The listing builds one solid part. Answer for the finished solid, in the listing's coordinates (mm). Face numbers are marked on the shaded views. A direction names the side the tool comes from. Give positions to 0.01 mm unless a question says otherwise; leave off trailing zeros. Loops run counter-clockwise (first coordinate to the right, second up) from the corner with the lowest first, then second, coordinate; pieces in that order, holes last. Notation, with made-up numbers: M 56,2 L 112,2 A26 cw 112,27 Z; hole C 87,72.5 d10. An arc over 180 degrees is marked long. Return JSON: item names as keys, results as strings.
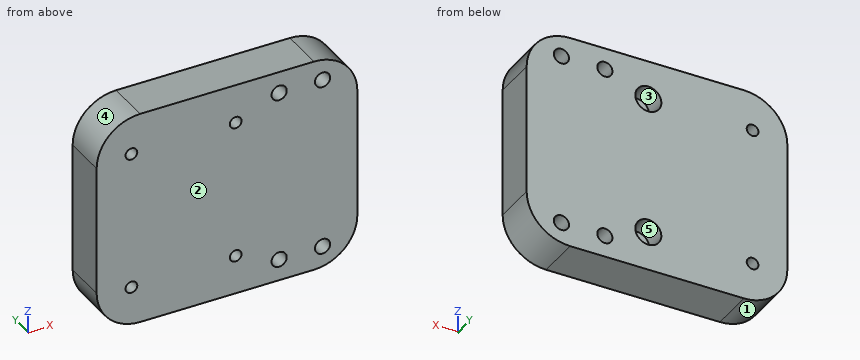
from build123d import *

# Parameters (mm, degrees)
SKETCH1_W           = 60
SKETCH1_H           = 50
BOSS_EXTRUDE1_DEPTH = 10
SKETCH2_R           = 1.35
CUT_EXTRUDE1_DEPTH  = 79.74007874
SKETCH3_R           = 1.75
CUT_EXTRUDE2_DEPTH  = 79.74007874
FILLET1_R           = 10
SKETCH4_R           = 3
CUT_EXTRUDE3_DEPTH  = 5


with BuildPart() as part:
    # Sketch1 → Boss-Extrude1 (new body)
    with BuildSketch(Plane(origin=(0, 0, 0), x_dir=(1, 0, 0), z_dir=(0, 1, 0))):
        with Locations((30, 25)):
            Rectangle(SKETCH1_W, SKETCH1_H)
    extrude(amount=BOSS_EXTRUDE1_DEPTH)

    # Sketch2 → Cut-Extrude1 (cut, through all)
    with BuildSketch(Plane(origin=(0, 10, 0), x_dir=(1, 0, 0), z_dir=(0, 1, 0))):
        with Locations(Location((8, 41, 0), (0, 0, 270))):
            Circle(SKETCH2_R)
        with Locations(Location((8, 9, 0), (0, 0, 270))):
            Circle(SKETCH2_R)
        with Locations(Location((32, 9, 0), (0, 0, 270))):
            Circle(SKETCH2_R)
        with Locations(Location((32, 41, 0), (0, 0, 270))):
            Circle(SKETCH2_R)
    extrude(amount=-CUT_EXTRUDE1_DEPTH, mode=Mode.SUBTRACT)

    # Sketch3 → Cut-Extrude2 (cut, through all)
    with BuildSketch(Plane(origin=(0, 10, 0), x_dir=(1, 0, 0), z_dir=(0, 1, 0))):
        with Locations(Location((42, 45, 0), (0, 0, 270))):
            Circle(SKETCH3_R)
        with Locations(Location((52, 45, 0), (0, 0, 270))):
            Circle(SKETCH3_R)
        with Locations(Location((52, 5, 0), (0, 0, 270))):
            Circle(SKETCH3_R)
        with Locations(Location((42, 5, 0), (0, 0, 270))):
            Circle(SKETCH3_R)
    extrude(amount=-CUT_EXTRUDE2_DEPTH, mode=Mode.SUBTRACT)

    # Fillet1
    fillet1_edges = [part.edges().sort_by_distance(p)[0] for p in [
        (0, 5, -50),
        (60, 5, -50),
        (60, 5, 0),
        (0, 5, 0),
    ]]
    fillet(fillet1_edges, radius=FILLET1_R)

    # Sketch4 → Cut-Extrude3 (cut)
    with BuildSketch(Plane(origin=(0, 10, 0), x_dir=(1, 0, 0), z_dir=(0, 1, 0))):
        with Locations(Location((32, 41, 0), (0, 0, 270))):
            Circle(SKETCH4_R)
        with Locations(Location((32, 9, 0), (0, 0, 270))):
            Circle(SKETCH4_R)
    extrude(amount=-CUT_EXTRUDE3_DEPTH, mode=Mode.SUBTRACT)


solid = part.part
(1) Straight lines are drawn through the part: line 1 along X through (y, z) = (5, -45); line 2 along X through (y, z) = (2.5, -9); line 3 along Z through (x, y) = (53, 1). For each, find the intervals that lie inside material, in ascending order.
Values follow:
{"line 1": "1.34 to 40.25, 43.75 to 50.25, 53.75 to 58.66", "line 2": "0.05 to 6.65, 9.35 to 30.65, 33.35 to 59.95", "line 3": "-49.54 to -46.44, -43.56 to -6.44, -3.56 to -0.46"}
(2) A tool of negligible diameter and unlimited length cuts with its end or side. For the marked faces 4 and 5, from which of +Z, -Z, +X, -X, +Y, -Y can it reach the whole face along a straight path? Write none if from no direction.
Values follow:
{"face 4": "+Z, -X, +Y, -Y", "face 5": "+Y"}
(3) Given pin 1 (3.5 mm diameter, centred on x = 32, z = -41, fed in from +Y); pin 2 (1.6 mm diameter, centred on x = 8, z = -9, fed in from -Y); pin 3 (4 mm diameter, centred on x = 6.5, y = 1, fed in from +Z), each flat-ended and moving along its own axis, determine where each tip first touches the part or whether it passes through.
Values follow:
{"pin 1": "y = 5", "pin 2": "through", "pin 3": "z = -0.11"}
(4) Determine the mould class of the marked faces 1, 2 and 3 for opening direction X: released by +X, released by -X, zero draft, split by the parting line, or undercut.
Values follow:
{"face 1": "released by -X", "face 2": "zero draft", "face 3": "undercut"}
(5) The part is cut by section C-C (y = 8.75). Give the number of separate pieces and of enclosed holes in the cut face, and give its area (3 significant figures).
Values follow:
{"separate pieces": "1", "enclosed holes": "8", "area": "2,810 mm²"}
(6) The part is cut by section A-A (x = 32). Determine the outline of the cut face in (y, z).
Values follow:
{"outline": "M 0,-50 L 10,-50 L 10,-44 L 5,-44 L 5,-42.35 L 0,-42.35 Z; M 0,-39.65 L 5,-39.65 L 5,-38 L 10,-38 L 10,-12 L 5,-12 L 5,-10.35 L 0,-10.35 Z; M 0,-7.65 L 5,-7.65 L 5,-6 L 10,-6 L 10,0 L 0,0 Z"}
(7) The part is cut by section D-D (z = -11). Determine the outline of the cut face in (x, y).
Values follow:
{"outline": "M 0,0 L 60,0 L 60,10 L 34.24,10 L 34.24,5 L 29.76,5 L 29.76,10 L 0,10 Z"}
(8) The part is cut by section B-B (z = -5). Determine the outline of the cut face in (x, y).
Values follow:
{"outline": "M 1.34,0 L 40.25,0 L 40.25,10 L 1.34,10 Z; M 43.75,0 L 50.25,0 L 50.25,10 L 43.75,10 Z; M 53.75,0 L 58.66,0 L 58.66,10 L 53.75,10 Z"}
